```python
from build123d import *

# Parameters (mm, degrees)
F0_R     = 16.4
F1_DEPTH = 61.5
F2_R     = 1.5
F3_DEPTH = 7.7
F4_R     = 4.25
F5_DEPTH = 1.7
F6_W     = 8.9
F6_H     = 1.5
F7_DEPTH = 7.2
F9_DEPTH = 1.5


with BuildPart() as f1:
    # F0 (on Top) → F1 (new body)
    with BuildSketch(Plane.XY):
        Circle(F0_R)
    extrude(amount=F1_DEPTH)

    # F2 (on face) → F3 (join)
    with BuildSketch(Plane.XY.offset(61.5)):
        Circle(F2_R)
    extrude(amount=F3_DEPTH)

    # F4 (on face) → F5 (join)
    with BuildSketch(Plane.XY.offset(61.5)):
        Circle(F4_R)
    extrude(amount=F5_DEPTH)

    # F6 (on face) → F7 (join)
    with BuildSketch(Plane.XY.offset(61.5)):
        with Locations((0, -11.93791)):
            Rectangle(F6_W, F6_H)
    extrude(amount=F7_DEPTH)

    # F8 (on face) → F9 (cut, through all)
    with BuildSketch(Plane.XZ.offset(12.68791)):
        Polygon((-4.45, 65.3), (-4.1, 68.7), (-4.45, 68.7), align=None)
        Polygon((-0.95, 65.3), (-0.6, 68.7), (-2.9, 68.7), (-2.55, 65.3), align=None)
        Polygon((2.9, 68.7), (0.6, 68.7), (0.95, 65.3), (2.55, 65.3), align=None)
        Polygon((4.45, 68.7), (4.1, 68.7), (4.45, 65.3), align=None)
    extrude(amount=-F9_DEPTH, mode=Mode.SUBTRACT)


solid = f1.part
```
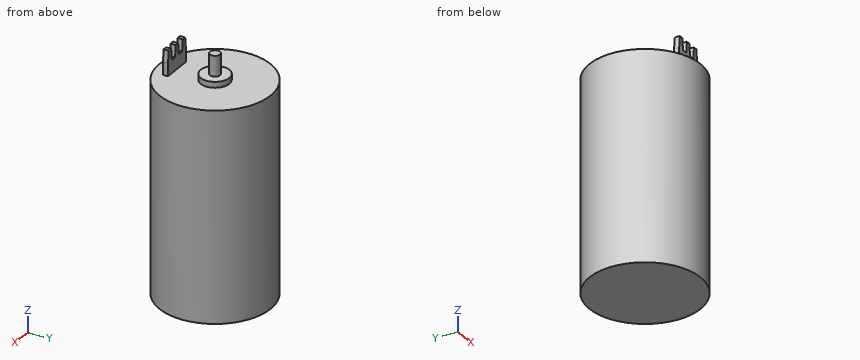
CAD build for the part. Positions are in the model's coordinates, mm. Round coordinates to 2 decimals unless told otherwise and drop trailing zeros. Order: outer loops, then holes, each group sorted by start corner. A loop starts at its lowest first (then second) coordinate and runs counter-clockwise, first axis right, second up.
Q1. Wall check: L1, parallel to Z at x = 10, y = -9; L2, parallel to Y at x = 5.5, z = 38; L3, parallel to X at y = -9.5, z = 51. Give the ranges that are in metal, low to high.
Q2. Drop flat-ended pins along their axis: pin 1 (0.6 mm diameter, centred on x = 3.5, y = -12, fed in from +Z); pin 2 (1 mm diameter, centred on y = 2.5, z = 34.5, fed in from +X); pin 3 (3.5 mm diameter, centred on x = 0, z = 65, fed in from +Y); pin 4 (1.5 mm diameter, centred on y = 0.5, z = 26, fed in from -X). Give the stop position or say it passes through.
Q3. Slice it at D-D (y = 6). Write the cut outline in (x, z).
Q4. Slice it at C-C (y = -9). Write the cut outline in (x, z).
Q5. Slice it at B-B (z = 33). Write the cut outline in (x, y).
Q6. Slice it at A-A (y = 0). Write the cut outline in (x, z), and give its area (3 significant figures).
Results below:
1. L1: z = 0 to 61.5
1. L2: y = -15.45 to 15.45
1. L3: x = -13.37 to 13.37
2. pin 1: stops at z = 68.7
2. pin 2: stops at x = 16.28
2. pin 3: stops at y = 1.5
2. pin 4: stops at x = -16.4
3. outline: (-15.26, 0) - (15.26, 0) - (15.26, 61.5) - (-15.26, 61.5) - close
4. outline: (-13.71, 0) - (13.71, 0) - (13.71, 61.5) - (-13.71, 61.5) - close
5. outline: circle Ø32.8 at (0, 0)
6. outline: (-16.4, 0) - (16.4, 0) - (16.4, 61.5) - (4.25, 61.5) - (4.25, 63.2) - (1.5, 63.2) - (1.5, 69.2) - (-1.5, 69.2) - (-1.5, 63.2) - (-4.25, 63.2) - (-4.25, 61.5) - (-16.4, 61.5) - close
6. area: 2,050 mm2
